from build123d import *

# Parameters (mm, degrees)
F0_W     = 76.2
F0_H     = 101.6
F1_DEPTH = 152.4
F3_DEPTH = 50.8
F4_R     = 5.5188922036


# Not quite as in the source:
# - a feature names something its author has since deleted; it is built from what else it names


with BuildPart() as f1:
    # F0 (on Top) → F1 (new body)
    with BuildSketch(Plane.XY):
        with Locations((-5.2541131154, 53.4473587833)):
            Rectangle(F0_W, F0_H)
    extrude(amount=-F1_DEPTH)

    # F2 (on face) → F3 (cut)
    with BuildSketch(Plane.YZ.offset(32.8458868846)):
        Polygon((15.3492157235, -137.4566919493), (91.5473587833, -137.988663984), (91.5473587833, -112.0566919493), (15.3492157235, -112.0566919493), align=None)
        Polygon((15.3492157235, -78.7826919493), (15.3492157235, -104.1826919493), (91.5473587833, -104.714663984), (91.5473587833, -78.7826919493), align=None)
        Polygon((15.3492157235, -45.5086919493), (15.3492157235, -70.9086919493), (91.5473587833, -71.440663984), (91.5473587833, -45.5086919493), align=None)
        Polygon((15.3492157235, -12.2346919493), (15.3492157235, -37.6346919493), (91.5473587833, -38.166663984), (91.5473587833, -12.2346919493), align=None)
    extrude(amount=-F3_DEPTH, mode=Mode.SUBTRACT)

    # F4
    f4_edges = [f1.edges().sort_by_distance(p)[0] for p in [
        (-5.254113, 104.247359, 0),
        (-5.254113, 2.647359, 0),
        (-5.254113, 2.647359, -152.4),
        (-5.254113, 104.247359, -152.4),
        (32.845887, 2.647359, -76.2),
        (32.845887, 53.447359, -152.4),
        (32.845887, 104.247359, -76.2),
        (-43.354113, 53.447359, -152.4),
        (-43.354113, 2.647359, -76.2),
        (32.845887, 53.447359, 0),
        (-43.354113, 53.447359, 0),
        (-43.354113, 104.247359, -76.2),
    ]]
    fillet(f4_edges, radius=F4_R)


solid = f1.part
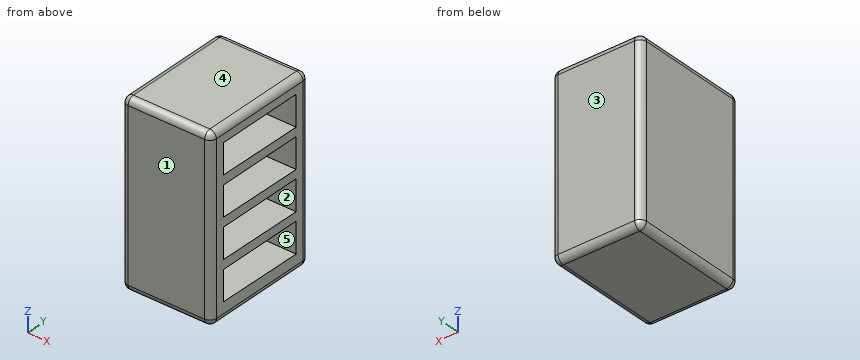
Geometry: final body of the model. Coordinates: model frame, mm. Face numbers are marked on the shaded views. A direction names the side the tool comes from. Round coordinates to 2 decimals unless told otherwise and drop trailing zeros. Loops run counter-clockwise (first coordinate to the right, second up) from the corner with the lowest first, then second, coordinate; pieces in that order, holes last. Notation, with made-up numbers: M 22,-3.5 L 62,-3.5 A9 cw 62,5.5 Z; hole C -0.5,44 d6. An arc over 180 degrees is marked long. One line per question, with ' | ' between items.
(1) Access query for the marked faces 1 and 2. Directions: +Z, -Z, +X, -X, +Y, -Y. A direction counts if a zero-diameter tool reaches every point of the face in a straight line with its end or side. Return the directions, or none.
Check result:
face 1: +Z, -Z, +X, -X, -Y | face 2: +X
(2) Contact query for a flat-ended pin moving along its axis: P1, Ø4, axis at y = 87, z = -94, coming from the +X side. Output: stop coordinate, or through.
Check result:
P1: stops at x = -17.95
(3) Cut plane D-D on y = 24. Return the cut outline in (x, z), plus the area to 3 significant figures.
Check result:
outline: M -43.35,-146.88 A5.52 ccw -37.84,-152.4 L 27.33,-152.4 A5.52 ccw 32.85,-146.88 L 32.85,-137.52 L -17.95,-137.52 L -17.95,-112.06 L 32.85,-112.06 L 32.85,-104.24 L -17.95,-104.24 L -17.95,-78.78 L 32.85,-78.78 L 32.85,-70.97 L -17.95,-70.97 L -17.95,-45.51 L 32.85,-45.51 L 32.85,-37.7 L -17.95,-37.7 L -17.95,-12.23 L 32.85,-12.23 L 32.85,-5.52 A5.52 ccw 27.33,0 L -37.84,0 A5.52 ccw -43.35,-5.52 Z | area: 6,410 mm2
(4) Cut plane C-C on y = 59. Return the cut outline in (x, z), plus the area to 3 significant figures.
Check result:
outline: M -43.35,-146.88 A5.52 ccw -37.84,-152.4 L 27.33,-152.4 A5.52 ccw 32.85,-146.88 L 32.85,-137.76 L -17.95,-137.76 L -17.95,-112.06 L 32.85,-112.06 L 32.85,-104.49 L -17.95,-104.49 L -17.95,-78.78 L 32.85,-78.78 L 32.85,-71.21 L -17.95,-71.21 L -17.95,-45.51 L 32.85,-45.51 L 32.85,-37.94 L -17.95,-37.94 L -17.95,-12.23 L 32.85,-12.23 L 32.85,-5.52 A5.52 ccw 27.33,0 L -37.84,0 A5.52 ccw -43.35,-5.52 Z | area: 6,360 mm2
(5) Cut plane A-A on x = 1. Return the cut outline in (y, z), plus the area to 3 significant figures.
Check result:
outline: M 2.65,-146.88 A5.52 ccw 8.17,-152.4 L 98.73,-152.4 A5.52 ccw 104.25,-146.88 L 104.25,-5.52 A5.52 ccw 98.73,0 L 8.17,0 A5.52 ccw 2.65,-5.52 Z; hole M 15.35,-137.46 L 91.55,-137.99 L 91.55,-112.06 L 15.35,-112.06 Z; hole M 15.35,-104.18 L 91.55,-104.71 L 91.55,-78.78 L 15.35,-78.78 Z; hole M 15.35,-70.91 L 91.55,-71.44 L 91.55,-45.51 L 15.35,-45.51 Z; hole M 15.35,-37.63 L 91.55,-38.17 L 91.55,-12.23 L 15.35,-12.23 Z | area: 7,630 mm2
(6) Material intervals for line 1 along Z through (x, y) = (-13, 88); line 2 along Y through (x, z) = (7, -90); line 3 along Z through (x, y) = (11.5, 73.5), sorted ascending. Write a range as from..to.
Check result:
line 1: z = -152.4..-137.96, -112.06..-104.69, -78.78..-71.42, -45.51..-38.14, -12.23..0 | line 2: y = 2.65..15.35, 91.55..104.25 | line 3: z = -152.4..-137.86, -112.06..-104.59, -78.78..-71.31, -45.51..-38.04, -12.23..0
(7) Pull-direction query (Z, two-part tool) for the marked faces 3, 4 and 5; classes: +Z half, -Z half, draft (parallel to the pull), parting line (faces both ways), or undercut.
Check result:
face 3: draft | face 4: +Z half | face 5: undercut
(8) Cut plane B-B on z = -28. Return the cut outline in (x, y), plus the area to 3 significant figures.
Check result:
outline: M -43.35,8.17 A5.52 ccw -37.84,2.65 L 27.33,2.65 A5.52 ccw 32.85,8.17 L 32.85,15.35 L -17.95,15.35 L -17.95,91.55 L 32.85,91.55 L 32.85,98.73 A5.52 ccw 27.33,104.25 L -37.84,104.25 A5.52 ccw -43.35,98.73 Z | area: 3,840 mm2
